Can you work these out from the model? Positions are in its coordinate system, mm. Face numbers are marked on the shaded views. A direction names the side the tool comes from. Give positions to 0.01 mm unless a question says otherwise; leave off trailing zeros. Order: outer loops, then holes, each group sorted by start corner. A loop starts at its lowest first (then second) coordinate and runs counter-clockwise, first axis right, second up. Notation, with made-up numbers: (56, -6.5) -> (92, -6.5) arc R31 cw to (92, 27.5) -> close; hole circle Ø6 at (7.5, -16). An arc over 180 degrees is marked (long way). Answer as CSV lines item,"result".
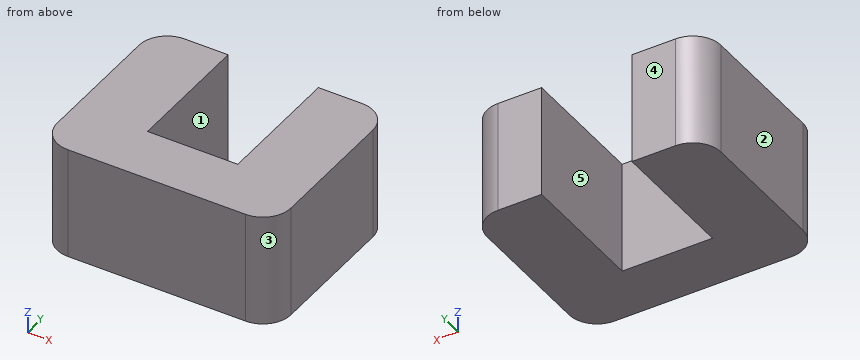
```python
from build123d import *

# Parameters (mm, degrees)
F1_DEPTH = 50.8


with BuildPart() as f1:
    # F0 (on Top) → F1 (new body)
    with BuildSketch(Plane.XY):
        with BuildLine():
            Line((-20.421574, 42.61367), (-40.162275, 42.61367))
            ThreePointArc((-40.162275, 42.61367), (-49.142532, 38.893926), (-52.862275, 29.91367))
            Line((-52.862275, 29.91367), (-52.862275, -29.91367))
            ThreePointArc((-52.862275, -29.91367), (-49.142532, -38.893926), (-40.162275, -42.61367))
            Line((-40.162275, -42.61367), (40.162275, -42.61367))
            ThreePointArc((40.162275, -42.61367), (49.142532, -38.893926), (52.862275, -29.91367))
            Line((52.862275, -29.91367), (52.862275, 29.91367))
            ThreePointArc((52.862275, 29.91367), (49.142532, 38.893926), (40.162275, 42.61367))
            Line((40.162275, 42.61367), (20.421574, 42.61367))
            Line((20.421574, 42.61367), (20.421574, -16.341066))
            Line((20.421574, -16.341066), (-20.421574, -16.341066))
            Line((-20.421574, -16.341066), (-20.421574, 42.61367))
        make_face()
    extrude(amount=F1_DEPTH)


solid = f1.part
```
Item 1: For pin 1 (5 mm diameter, centred on x = 0.5, z = 42.5, fed in from +Y), with a flat end and sliding along its axis, tell me the tip position at first contact or that it passes through.
Numbers:
pin 1,"stops at y = -16.34"
Item 2: Imagine slicing it at B-B, the plane z = 18. Please give me the cut outline in (x, y), then the cut area to 3 significant figures.
Numbers:
outline,"(-52.86, -29.91) arc R12.7 ccw to (-40.16, -42.61) -> (40.16, -42.61) arc R12.7 ccw to (52.86, -29.91) -> (52.86, 29.91) arc R12.7 ccw to (40.16, 42.61) -> (20.42, 42.61) -> (20.42, -16.34) -> (-20.42, -16.34) -> (-20.42, 42.61) -> (-40.16, 42.61) arc R12.7 ccw to (-52.86, 29.91) -> close"
area,"6,460 mm²"
Item 3: Please list where these lines run through material, in increasing order: line 1 along X through (y, z) = (30.5, 23.5); line 2 along X through (y, z) = (-10, 46); line 3 along Y through (x, z) = (17, 5).
Numbers:
line 1,"x = -52.85 to -20.42, 20.42 to 52.85"
line 2,"x = -52.86 to -20.42, 20.42 to 52.86"
line 3,"y = -42.61 to -16.34"
Item 4: Imagine slicing it at D-D, the plane y = 37. Please give me the cut outline in (x, z), then the cut area to 3 significant figures.
Numbers:
outline,"(-50.7, 0) -> (-20.42, 0) -> (-20.42, 50.8) -> (-50.7, 50.8) -> close; (20.42, 0) -> (50.7, 0) -> (50.7, 50.8) -> (20.42, 50.8) -> close"
area,"3,080 mm²"
Item 5: For the marked faces 4 and 5, which set-ups out of +Z, -Z, +X, -X, +Y, -Y let a thin tool reach every point of the face, with its end or its side?
Numbers:
face 4,"+Z, -Z, +X, -X, +Y"
face 5,"+Z, -Z, +Y"
Item 6: We'd pull the mould along X, two halves only. Please class the marked faces 1, 2 and 3: released by +X, released by -X, zero draft, split by the parting line, or undercut.
Numbers:
face 1,"undercut"
face 2,"released by -X"
face 3,"released by +X"
Item 7: Imagine slicing it at A-A, the plane y = 23. Please give me the cut outline in (x, z), then the cut area to 3 significant figures.
Numbers:
outline,"(-52.86, 0) -> (-20.42, 0) -> (-20.42, 50.8) -> (-52.86, 50.8) -> close; (20.42, 0) -> (52.86, 0) -> (52.86, 50.8) -> (20.42, 50.8) -> close"
area,"3,300 mm²"
Item 8: Imagine slicing it at C-C, the plane x = 18.5. Please give me the cut outline in (y, z), then the cut area to 3 significant figures.
Numbers:
outline,"(-42.61, 0) -> (-16.34, 0) -> (-16.34, 50.8) -> (-42.61, 50.8) -> close"
area,"1,330 mm²"
